The model under review builds one solid part; all positions refer to its coordinate system, in mm. Give positions to 0.01 mm unless a question says otherwise; leave off trailing zeros.
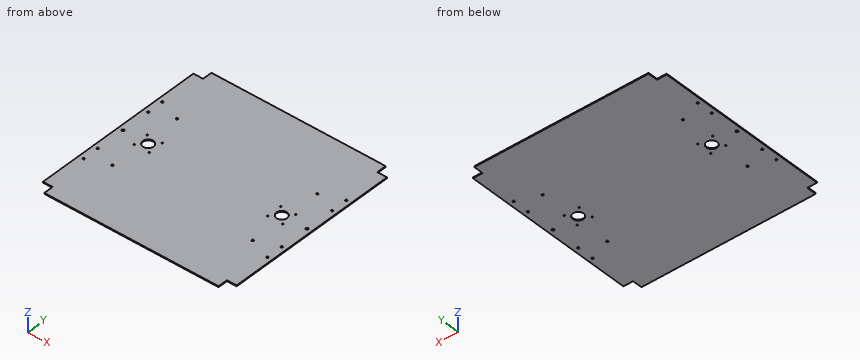
```python
from build123d import *

# Parameters (mm, degrees)
F0_R     = 2
F0_R_2   = 1.5
F0_R_3   = 2.5
F0_R_4   = 11
F1_DEPTH = 2


with BuildPart() as f1:
    # F0 (on Top) → F1 (new body)
    with BuildSketch(Plane.XY):
        Polygon((200, -180), (200, 180), (180, 180), (180, 200), (-180, 200), (-180, 180), (-200, 180), (-200, -180), (-180, -180), (-180, -200), (180, -200), (180, -180), align=None)
        with Locations((-190.000003, -94.5)):
            Circle(F0_R, mode=Mode.SUBTRACT)
        with Locations((-190.000003, -60.5)):
            Circle(F0_R, mode=Mode.SUBTRACT)
        with Locations((-145.000003, -77.5)):
            Circle(F0_R, mode=Mode.SUBTRACT)
        with Locations((-153.5, -15.5)):
            Circle(F0_R_2, mode=Mode.SUBTRACT)
        with Locations((-122.5, -15.5)):
            Circle(F0_R_2, mode=Mode.SUBTRACT)
        with Locations((145.000003, -77.5)):
            Circle(F0_R, mode=Mode.SUBTRACT)
        with Locations((190.000003, -94.5)):
            Circle(F0_R, mode=Mode.SUBTRACT)
        with Locations((190.000003, -60.5)):
            Circle(F0_R, mode=Mode.SUBTRACT)
        with Locations((122.5, -15.5)):
            Circle(F0_R_2, mode=Mode.SUBTRACT)
        with Locations((153.5, -15.5)):
            Circle(F0_R_2, mode=Mode.SUBTRACT)
        with Locations((-190, 0)):
            Circle(F0_R_3, mode=Mode.SUBTRACT)
        with Locations((-153.5, 15.5)):
            Circle(F0_R_2, mode=Mode.SUBTRACT)
        with Locations((-138, 0)):
            Circle(F0_R_4, mode=Mode.SUBTRACT)
        with Locations((-122.5, 15.5)):
            Circle(F0_R_2, mode=Mode.SUBTRACT)
        with Locations((-190, 60.199966)):
            Circle(F0_R, mode=Mode.SUBTRACT)
        with Locations((-190, 94.199966)):
            Circle(F0_R, mode=Mode.SUBTRACT)
        with Locations((-145, 77.199966)):
            Circle(F0_R, mode=Mode.SUBTRACT)
        with Locations((122.5, 15.5)):
            Circle(F0_R_2, mode=Mode.SUBTRACT)
        with Locations((138, 0)):
            Circle(F0_R_4, mode=Mode.SUBTRACT)
        with Locations((153.5, 15.5)):
            Circle(F0_R_2, mode=Mode.SUBTRACT)
        with Locations((190, 0)):
            Circle(F0_R_3, mode=Mode.SUBTRACT)
        with Locations((145, 77.199966)):
            Circle(F0_R, mode=Mode.SUBTRACT)
        with Locations((190, 60.199966)):
            Circle(F0_R, mode=Mode.SUBTRACT)
        with Locations((190, 94.199966)):
            Circle(F0_R, mode=Mode.SUBTRACT)
    extrude(amount=-F1_DEPTH)


solid = f1.part
```
Item 1: For line 1 (X direction, y = -61, z = -0.3); line 2 (Y direction, x = 153.5, z = -1.5); line 3 (Y direction, x = 138, z = -0.6), list the stretches that pass through material, from the lowest coordinate up.
Values found:
line 1: x = -200 to -191.94, -188.06 to 188.06, 191.94 to 200
line 2: y = -200 to -17, -14 to 14, 17 to 200
line 3: y = -200 to -11, 11 to 200
Item 2: Take a section at A-A (z = -0.35). Give the number of separate pieces and of enclosed holes in the cut face, and give its area (3 significant figures).
Values found:
separate pieces: 1
enclosed holes: 24
area: 157,000 mm2
Item 3: Clearance check with flat-ended pins moving along their axes: pin 1 Ø0.6 at (y, z) = (187.5, -1) entering from -X; pin 2 Ø0.6 at (y, z) = (-185, -0.5) entering from +X; pin 3 Ø3 at (x, y) = (190, 60.2) entering from +Z. State where each tip first meets the part, or that it passes through.
Values found:
pin 1: stops at x = -180
pin 2: stops at x = 180
pin 3: passes through
